The model under review builds one solid part; all positions refer to its coordinate system, in mm. Face numbers are marked on the shaded views. A direction names the side the tool comes from. Coordinates: 2 decimals unless noted, no trailing zeros. Order: outer loops, then holes, each group sorted by start corner. A loop starts at its lowest first (then second) coordinate and runs counter-clockwise, first axis right, second up. Notation, with made-up numbers: (20, 86.5) -> (36, 86.5) arc R27 cw to (36, 117.5) -> close; hole circle Ø10 at (-3, 4). An arc over 180 degrees is marked (long way). Put each result on its own line as item: value.
from build123d import *

# Parameters (mm, degrees)
F_01_START                                     = -1.65
S01_ISO_7380_BUTTON_HEAD_CLEARANCE_ENV_R       = 2.85
F_01_ISO_7380_BUTTON_HEAD_CLEARANCE_ENVE_DEPTH = 1.65
S02_M3_UNDERHEAD_LENGTH_R                      = 1.5
F_02_M3_UNDERHEAD_LENGTH_DEPTH                 = 6
F_03_START                                     = -1.75
F_03_BUTTON_HEAD_HEX_SOCKET_DEPTH              = 1.12


with BuildPart() as part:
    # S01 - ISO 7380 button head clearance envelope → 01 - ISO 7380 button head clearance envelope (new body)
    with BuildSketch(Plane.XY.offset(F_01_START)):
        Circle(S01_ISO_7380_BUTTON_HEAD_CLEARANCE_ENV_R)
    extrude(amount=F_01_ISO_7380_BUTTON_HEAD_CLEARANCE_ENVE_DEPTH)

    # S02 - M3 underhead length → 02 - M3 underhead length (add)
    with BuildSketch(Plane.XY):
        Circle(S02_M3_UNDERHEAD_LENGTH_R)
    extrude(amount=F_02_M3_UNDERHEAD_LENGTH_DEPTH)

    # S03 - Button head hex socket → 03 - Button head hex socket (cut)
    with BuildSketch(Plane.XY.offset(F_03_START)):
        Polygon((1.154700538, 0), (0.577350269, 1), (-0.577350269, 1), (-1.154700538, 0), (-0.577350269, -1), (0.577350269, -1), align=None)
    extrude(amount=F_03_BUTTON_HEAD_HEX_SOCKET_DEPTH, mode=Mode.SUBTRACT)


solid = part.part
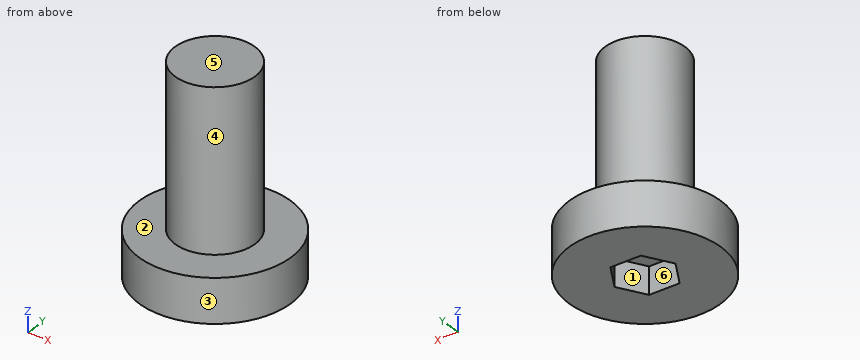
Item 1: Consider section C-C on y = -1.1. Write out the cut boundary in (x, z), and give its area (3 significant figures).
Answers below:
outline: (-2.63, -1.65) -> (2.63, -1.65) -> (2.63, 0) -> (1.02, 0) -> (1.02, 6) -> (-1.02, 6) -> (-1.02, 0) -> (-2.63, 0) -> close
area: 20.9 mm^2
Item 2: For pin 1 Ø1.5 at (x, z) = (-1.5, 0.5) entering from -Y; pin 2 Ø3 at (x, z) = (-2.5, 0) entering from +Y; pin 3 Ø1 at (x, z) = (-1.5, 3.5) entering from -Y, all flat-tipped, find the tip position at first contact; note any pin that passes through.
Answers below:
pin 1: y = -2.69
pin 2: y = 2.67
pin 3: y = -1.12
Item 3: Mouldability with a two-part tool opening along X and no side actions: class the marked faces 1, 2 and 3 as +X half, -X half, draft (parallel to the pull), parting line (faces both ways), or undercut.
Answers below:
face 1: undercut
face 2: draft
face 3: parting line
Item 4: Consider section A-A on z = -0.75. Write out the cut boundary in (x, y), and give its area (3 significant figures).
Answers below:
outline: circle Ø5.7 at (0, 0); hole (-1.15, 0) -> (-0.58, -1) -> (0.58, -1) -> (1.15, 0) -> (0.58, 1) -> (-0.58, 1) -> close
area: 22.1 mm^2
Item 5: Consider section B-B on x = 0. Write out the cut boundary in (y, z).
Answers below:
outline: (-2.85, -1.65) -> (-1, -1.65) -> (-1, -0.63) -> (1, -0.63) -> (1, -1.65) -> (2.85, -1.65) -> (2.85, 0) -> (1.5, 0) -> (1.5, 6) -> (-1.5, 6) -> (-1.5, 0) -> (-2.85, 0) -> close
Item 6: For the marked faces 4, 5 and 6, list the 3-axis set-ups (+Z, -Z, +X, -X, +Y, -Y) from which the entire face can be reached by the end or side of a thin tool; tool diameter is ignored.
Answers below:
face 4: +Z
face 5: +Z, +X, -X, +Y, -Y
face 6: -Z
Item 7: Consider section D-D on z = 1. Write out the cut boundary in (x, y).
Answers below:
outline: circle Ø3 at (0, 0)
Item 8: For line 1 (Z direction, x = -2.45, y = 0.6); line 2 (X direction, y = -0.05, z = -0.75); line 3 (X direction, y = 0.5, z = 5.25), list the stretches that pass through material, from the lowest coordinate up. Write a range as from..to.
Answers below:
line 1: -1.65..0
line 2: -2.85..-1.13, 1.13..2.85
line 3: -1.41..1.41
